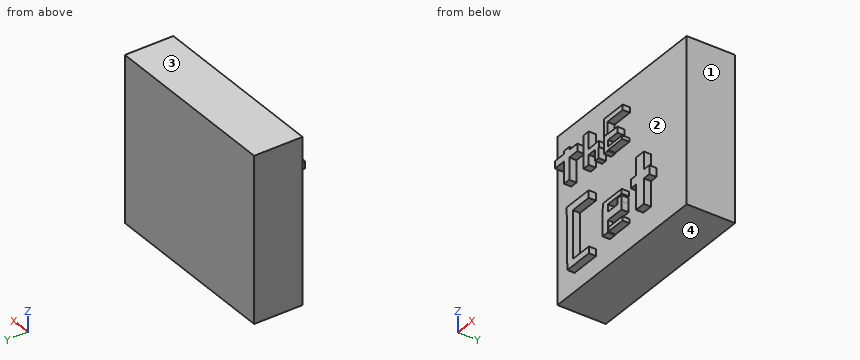
```python
from build123d import *

# Parameters (mm, degrees)
F0_W      = 95.87875
F0_H      = 86.435549
F1_DEPTH  = 25.4
F2_W      = 3.831741
F2_H      = 16.888321
F22_DEPTH = 3.81
F4_W      = 3.871451
F4_H      = 17.145001
F23_DEPTH = 3.81
F6_W      = 2.765321
F6_H      = 8.849032
F24_DEPTH = 3.81
F3_W      = 16.604224
F3_H      = 3.865305
F25_DEPTH = 3.81
F5_W      = 11.43
F5_H      = 2.949677
F26_DEPTH = 3.81
F7_W      = 10.047339
F7_H      = 3.134032
F27_DEPTH = 3.81
F21_W     = 13.642261
F21_H     = 4.60887
F28_DEPTH = 3.81
F20_W     = 5.715003
F20_H     = 26.915808
F29_DEPTH = 3.81
F19_W     = 10.508227
F19_H     = 2.21226
F30_DEPTH = 3.81
F18_W     = 10.139517
F18_H     = 4.240159
F31_DEPTH = 3.81
F17_W     = 3.041856
F17_H     = 3.50274
F32_DEPTH = 3.81
F16_W     = 13.826613
F16_H     = 2.396613
F33_DEPTH = 3.81
F15_W     = 3.871451
F15_H     = 14.379678
F34_DEPTH = 3.81
F14_W     = 16.038871
F14_H     = 3.502741
F35_DEPTH = 3.81
F8_W      = 3.134032
F8_H      = 8.849032
F36_DEPTH = 3.81
F9_W      = 13.457904
F9_H      = 1.843549
F37_DEPTH = 3.81
F10_W     = 2.580968
F10_H     = 8.480324
F38_DEPTH = 3.81
F11_W     = 13.826613
F11_H     = 2.765322
F39_DEPTH = 3.81
F12_W     = 4.424516
F12_H     = 29.128066
F40_DEPTH = 3.81
F13_W     = 16.40758
F13_H     = 3.871451
F41_DEPTH = 3.81


with BuildPart() as f1:
    # F0 (on Front) → F1 (new body)
    with BuildSketch(Plane.XZ):
        with Locations((-1.902111, -7.113785)):
            Rectangle(F0_W, F0_H)
    extrude(amount=F1_DEPTH)

    # F2 (on face) → F22 (join)
    with BuildSketch(Plane.XZ.offset(25.4)):
        with Locations((-37.61089, 13.43617)):
            Rectangle(F2_W, F2_H)
    extrude(amount=F22_DEPTH)

    # F4 (on face) → F23 (join)
    with BuildSketch(Plane.XZ.offset(25.4)):
        with Locations((-23.22871, 13.457904)):
            Rectangle(F4_W, F4_H)
    extrude(amount=F23_DEPTH)

    # F6 (on face) → F24 (join)
    with BuildSketch(Plane.XZ.offset(25.4)):
        with Locations((-15.301452, 8.756855)):
            Rectangle(F6_W, F6_H)
    extrude(amount=F24_DEPTH)

    # F3 (on face) → F25 (join)
    with BuildSketch(Plane.XZ.offset(25.4)):
        with Locations((-38.03664, 18.385231)):
            Rectangle(F3_W, F3_H)
    extrude(amount=F25_DEPTH)

    # F5 (on face) → F26 (join)
    with BuildSketch(Plane.XZ.offset(25.4)):
        with Locations((-19.449435, 11.522177)):
            Rectangle(F5_W, F5_H)
    extrude(amount=F26_DEPTH)

    # F7 (on face) → F27 (join)
    with BuildSketch(Plane.XZ.offset(25.4)):
        with Locations((-5.023669, 11.43)):
            Rectangle(F7_W, F7_H)
    extrude(amount=F27_DEPTH)

    # F21 (on face) → F28 (join)
    with BuildSketch(Plane.XZ.offset(25.4)):
        with Locations((16.868469, -21.938225)):
            Rectangle(F21_W, F21_H)
    extrude(amount=F28_DEPTH)

    # F20 (on face) → F29 (join)
    with BuildSketch(Plane.XZ.offset(25.4)):
        with Locations((16.77629, -23.873953)):
            Rectangle(F20_W, F20_H)
    extrude(amount=F29_DEPTH)

    # F19 (on face) → F30 (join)
    with BuildSketch(Plane.XZ.offset(25.4)):
        with Locations((-1.474838, -36.225727)):
            Rectangle(F19_W, F19_H)
    extrude(amount=F30_DEPTH)

    # F18 (on face) → F31 (join)
    with BuildSketch(Plane.XZ.offset(25.4)):
        with Locations((-2.027902, -29.128065)):
            Rectangle(F18_W, F18_H)
    extrude(amount=F31_DEPTH)

    # F17 (on face) → F32 (join)
    with BuildSketch(Plane.XZ.offset(25.4)):
        with Locations((1.520928, -25.625323)):
            Rectangle(F17_W, F17_H)
    extrude(amount=F32_DEPTH)

    # F16 (on face) → F33 (join)
    with BuildSketch(Plane.XZ.offset(25.4)):
        with Locations((-3.687095, -21.938226)):
            Rectangle(F16_W, F16_H)
    extrude(amount=F33_DEPTH)

    # F15 (on face) → F34 (join)
    with BuildSketch(Plane.XZ.offset(25.4)):
        with Locations((-9.033386, -30.326371)):
            Rectangle(F15_W, F15_H)
    extrude(amount=F34_DEPTH)

    # F14 (on face) → F35 (join)
    with BuildSketch(Plane.XZ.offset(25.4)):
        with Locations((-29.128065, -38.898871)):
            Rectangle(F14_W, F14_H)
    extrude(amount=F35_DEPTH)

    # F8 (on face) → F36 (join)
    with BuildSketch(Plane.XZ.offset(25.4)):
        with Locations((-8.480323, 8.756855)):
            Rectangle(F8_W, F8_H)
    extrude(amount=F36_DEPTH)

    # F9 (on face) → F37 (join)
    with BuildSketch(Plane.XZ.offset(25.4)):
        with Locations((-3.134032, 5.622822)):
            Rectangle(F9_W, F9_H)
    extrude(amount=F37_DEPTH)

    # F10 (on face) → F38 (join)
    with BuildSketch(Plane.XZ.offset(25.4)):
        with Locations((-8.756855, 17.605888)):
            Rectangle(F10_W, F10_H)
    extrude(amount=F38_DEPTH)

    # F11 (on face) → F39 (join)
    with BuildSketch(Plane.XZ.offset(25.4)):
        with Locations((-2.949677, 20.832096)):
            Rectangle(F11_W, F11_H)
    extrude(amount=F39_DEPTH)

    # F12 (on face) → F40 (join)
    with BuildSketch(Plane.XZ.offset(25.4)):
        with Locations((-35.303952, -22.767824)):
            Rectangle(F12_W, F12_H)
    extrude(amount=F40_DEPTH)

    # F13 (on face) → F41 (join)
    with BuildSketch(Plane.XZ.offset(25.4)):
        with Locations((-29.496774, -10.139516)):
            Rectangle(F13_W, F13_H)
    extrude(amount=F41_DEPTH)


solid = f1.part
```
Build history of the part. All positions in model axes, mm. Face numbers are marked on the shaded views. Coordinates: 2 decimals unless noted, no trailing zeros. Order: outer loops, then holes, each group sorted by start corner. A loop starts at its lowest first (then second) coordinate and runs counter-clockwise, first axis right, second up. Notation, with made-up numbers: (-22.5, -30.5) -> (10.5, -30.5) arc R21 cw to (10.5, -10.5) -> close; hole circle Ø10 at (48.5, 68). An arc over 180 degrees is marked (long way). Answer in a Markdown table with one row per item. Add a question column.
Q1. Mould opens along Z. For the marked faces 1, 2, 3 and 4 say: +Z half, -Z half, draft (parallel to the pull), parting line (faces both ways), or undercut.
Q2. Band-saw the part on A-A, the plane x = 21.5. List the corners of the cut face in (y, z).
Q3. Band-saw the part on B-B, the plane z = -16. List the corners of the cut face in (x, y).
Q4. Wall check: line 1 along Z through (x, y) = (-35.5, -27); line 2 along Y through (x, z) = (-22, 22.5). Give the ranges that are in metal, low to high. Write a range as [from, to].
Q5. Band-saw the part on D-D, the plane z = -28.5. List the corners of the cut face in (x, y).
Q6. Drop flat-ended pins along their axis: pin 1 (1.1 mm diameter, centred on x = -2, y = -27.5, fed in from -Z); pin 2 (2.5 mm diameter, centred on x = -8, y = -28, fed in from -Z); pin 3 (3 mm diameter, centred on x = -15, y = -28, fed in from +Z). Give the stop position or say it passes through.
Q7. Band-saw the part on C-C, the plane x = -42. List the corners of the cut face in (y, z).
Answers follow:
| question | item | result |
|---|---|---|
| 1 | face 1 | draft |
| 1 | face 2 | undercut |
| 1 | face 3 | +Z half |
| 1 | face 4 | -Z half |
| 2 | outline | (-29.21, -24.24) -> (-25.4, -24.24) -> (-25.4, -50.33) -> (0, -50.33) -> (0, 36.1) -> (-25.4, 36.1) -> (-25.4, -19.63) -> (-29.21, -19.63) -> close |
| 3 | outline | (-49.84, -25.4) -> (-37.52, -25.4) -> (-37.52, -29.21) -> (-33.09, -29.21) -> (-33.09, -25.4) -> (13.92, -25.4) -> (13.92, -29.21) -> (19.63, -29.21) -> (19.63, -25.4) -> (46.04, -25.4) -> (46.04, 0) -> (-49.84, 0) -> close |
| 4 | line 1 | [-40.65, -8.2], [16.45, 20.32] |
| 4 | line 2 | [-25.4, 0] |
| 5 | outline | (-49.84, -25.4) -> (-37.52, -25.4) -> (-37.52, -29.21) -> (-33.09, -29.21) -> (-33.09, -25.4) -> (-10.97, -25.4) -> (-10.97, -29.21) -> (3.04, -29.21) -> (3.04, -25.4) -> (13.92, -25.4) -> (13.92, -29.21) -> (19.63, -29.21) -> (19.63, -25.4) -> (46.04, -25.4) -> (46.04, 0) -> (-49.84, 0) -> close |
| 6 | pin 1 | z = -37.33 |
| 6 | pin 2 | z = -37.52 |
| 6 | pin 3 | z = 13.18 |
| 7 | outline | (-29.21, 16.45) -> (-25.4, 16.45) -> (-25.4, -50.33) -> (0, -50.33) -> (0, 36.1) -> (-25.4, 36.1) -> (-25.4, 20.32) -> (-29.21, 20.32) -> close |
